```python
from build123d import *

# Parameters (mm, degrees)
EXTRUDE_1_DEPTH = 10
SCALE_1_SCALE   = 0.2


with BuildPart() as part:
    # Эскиз1 → Бобышка-Вытянуть1 (new body)
    with BuildSketch(Plane.XY):
        with BuildLine():
            Line((-60, -45), (-27.583269132, -45))
            ThreePointArc((-27.583269132, -45), (-20.06001769, -64.277376125), (-5.945767968, -79.41027067))
            ThreePointArc((-5.945767968, -79.41027067), (-2.542345747, -82.680315027), (0, -86.656865167))
            Line((0, -86.656865167), (0, -19.711115149))
            ThreePointArc((0, -19.711115149), (-5.008387109, -15.151161707), (-11.091351129, -12.172124017))
            ThreePointArc((-11.091351129, -12.172124017), (-4.677676581, 0.965070873), (0, 14.815718966))
            Line((0, 14.815718966), (0, 113.343134833))
            ThreePointArc((0, 113.343134833), (-5.562430401, 104.106601718), (-7.5, 93.5))
            Line((-7.5, 93.5), (-5, 44.25))
            ThreePointArc((-5, 44.25), (-8.525159088, 17.271181236), (-18.863936417, -7.896120801))
            ThreePointArc((-18.863936417, -7.896120801), (-34.990467135, -0.436539144), (-19.576058944, 8.401241779))
            Line((-19.576058944, 8.401241779), (-22.449472465, 49.49296956))
            ThreePointArc((-22.449472465, 49.49296956), (-33.881518529, 82.214174393), (-60, 105))
            Line((-60, 105), (-60, -45))
        make_face()
        with BuildLine():
            ThreePointArc((-26.401072965, -19.950864506), (-27.972740949, -27.40259956), (-28.5, -35))
            Line((-28.5, -35), (-50, -35))
            Line((-50, -35), (-50, -5))
            Line((-50, -5), (-44.364916731, -5))
            ThreePointArc((-44.364916731, -5), (-37.794087282, -15.372421104), (-26.401072965, -19.950864506))
        make_face(mode=Mode.SUBTRACT)
        with BuildLine():
            Line((-5, -45), (-5, -67.136427928))
            ThreePointArc((-5, -67.136427928), (-12.779082294, -56.957998409), (-17.374821937, -45))
            Line((-17.374821937, -45), (-5, -45))
        make_face(mode=Mode.SUBTRACT)
        with BuildLine():
            Line((-4.5, -35), (-18.5, -35))
            ThreePointArc((-18.5, -35), (-17.952221542, -28), (-16.322222222, -21.170419965))
            ThreePointArc((-16.322222222, -21.170419965), (-7.858362699, -25.902991945), (-4.5, -35))
        make_face(mode=Mode.SUBTRACT)
        with BuildLine():
            Line((-44.364916731, 5), (-50, 5))
            Line((-50, 5), (-50, 85.909197079))
            ThreePointArc((-50, 85.909197079), (-37.591425702, 68.515820434), (-32.355603325, 47.801370616))
            Line((-32.355603325, 47.801370616), (-30.360374841, 19.268273964))
            ThreePointArc((-30.360374841, 19.268273964), (-39.273434111, 14.009606657), (-44.364916731, 5))
        make_face(mode=Mode.SUBTRACT)
    extrude_1 = extrude(amount=EXTRUDE_1_DEPTH)

    # Зеркальное отражение1: Бобышка-Вытянуть1 across plane
    add(extrude_1.mirror(Plane(origin=(0, 0, 0), x_dir=(0, 0, 1), z_dir=(1, 0, 0))))


with BuildPart() as part_1:
    # Масштаб1: scaled about (0, 12.329369983, 5)
    add(part.part.scale(SCALE_1_SCALE).moved(Location((0, 9.863495986, 4))))


solid = part_1.part
```
Could you check a few things on this model? Use its own coordinates, in mm. A direction names the side the tool comes from. Round coordinates to 2 decimals unless told otherwise and drop trailing zeros. Loops run counter-clockwise (first coordinate to the right, second up) from the corner with the lowest first, then second, coordinate; pieces in that order, holes last. Notation, with made-up numbers: (52, 5) -> (96, 5) arc R22 cw to (96, 26) -> close; hole circle Ø3 at (-31, -18). An arc over 180 degrees is marked (long way). One line per question, with ' | ' between items.
(1) If we section it at A-A on x = 8.25: List the corners of the cut face in (y, z) for me, and give its area (3 significant figures).
Model answer:
outline: (0.86, 4) -> (2.86, 4) -> (2.86, 6) -> (0.86, 6) -> close; (7.53, 4) -> (12.2, 4) -> (12.2, 6) -> (7.53, 6) -> close; (24.91, 4) -> (28.12, 4) -> (28.12, 6) -> (24.91, 6) -> close | area: 19.8 mm^2
(2) For faces 1 (the face through (6.274, 16.61, 4.986)), 2 (the face through (-4.043, -2.943, 4.986)), which set-ups out of +Z, -Z, +X, -X, +Y, -Y let a thin tool reach every point of the face, with its end or its side?
Model answer:
face 1: +Z, -Z | face 2: +Z, -Z, -X, -Y
(3) For pin 1 Ø1.2 at (x, z) = (-9, 5) entering from -Y; pin 2 Ø0.6 at (x, z) = (9.5, 5) entering from +Y; pin 3 Ø1.2 at (x, z) = (-9.5, 5.5) entering from +Y, each with a flat end and sliding along its axis, tell me the tip position at first contact or that it passes through.
Model answer:
pin 1: stops at y = 0.86 | pin 2: stops at y = 29.5 | pin 3: stops at y = 29.72
(4) If I drill on probe 1 along Y at (x, z) = (7.75, 4.25); probe 2 along X at (y, z) = (14, 4.2); probe 3 along X at (y, z) = (22.5, 4.2), over which ranges is the centre line in solid material (lowest first)?
Model answer:
probe 1: y = 0.86 to 2.86, 6.96 to 12.77, 24.04 to 27.58 | probe 2: x = -12 to -10, -6.09 to -4.09, -1.54 to 1.54, 4.09 to 6.09, 10 to 12 | probe 3: x = -12 to -10, -7.09 to -4.99, -1.19 to 1.19, 4.99 to 7.09, 10 to 12
(5) Thinking about a two-plate mould opening in X: for faces 3 (the face through (-0.95, 10.02, 4.99)), 4 (the face through (12, 16, 5)), 5 (the face through (-0.52, -6.66, 4.99)), 6 (the face through (-7.83, 12.69, 4.99)), which applies, released by +X, released by -X, zero draft, split by the parting line, or undercut?
Model answer:
face 3: undercut | face 4: released by +X | face 5: released by -X | face 6: undercut
(6) If we section it at B-B on y = 5: List the corners of the cut face in (x, z) for me.
Model answer:
outline: (-12, 4) -> (-10, 4) -> (-10, 6) -> (-12, 6) -> close; (-5.49, 4) -> (-3.44, 4) -> (-3.44, 6) -> (-5.49, 6) -> close; (-1.89, 4) -> (1.89, 4) -> (1.89, 6) -> (-1.89, 6) -> close; (3.44, 4) -> (5.49, 4) -> (5.49, 6) -> (3.44, 6) -> close; (10, 4) -> (12, 4) -> (12, 6) -> (10, 6) -> close
(7) If we section it at C-C on z = 4.75: Count the separate pieces of the cut face and the enclosed holes in it, and give its area (3 significant figures).
Model answer:
separate pieces: 1 | enclosed holes: 9 | area: 415 mm^2
